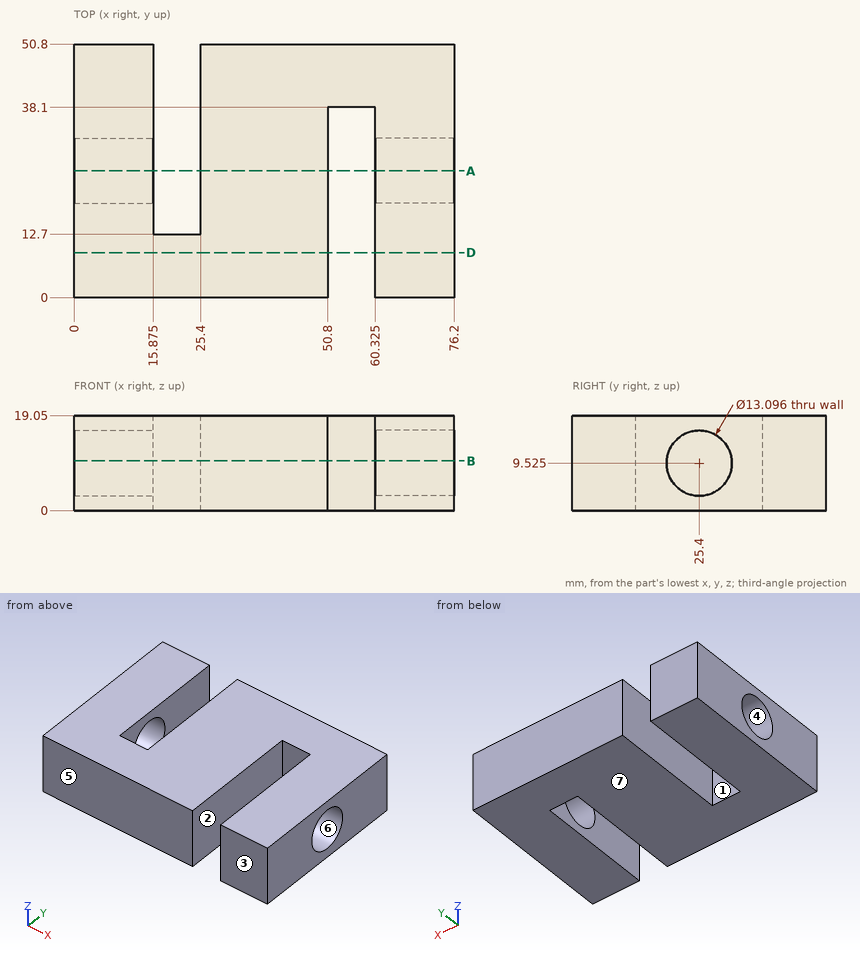
Verification items for this drawing (mm, ordinates from the low corner). A direction names the side the tool comes from. Give positions to 0.01 mm unless a question says otherwise; leave off trailing zeros. Write each loop counter-clockwise with the first axis right and the second up, starting at its lowest first coordinate (ties: lowest second). Pieces come first, ordered by that corner, then holes. Notation, with made-up numbers: M -26,-0.75 L 33,-0.75 A5 cw 33,8.25 Z; hole C 40.5,3.5 d3. An arc over 180 degrees is marked long. Use one line per item in the form item = value.
(1) Tool access check on the marked faces 1, 2 and 3. Record the directions out of +Z, -Z, +X, -X, +Y, -Y that give a thin tool (end or side, any length) a straight path to the whole face; none if there is none.
Answer block:
face_1 = +Z, -Z, +Y
face_2 = +Z, -Z, -Y
face_3 = +Z, -Z, +X, -X, -Y
(2) Section check D-D on y = 9. Record the boundary of the cut face in (x, z) (3 decimals).
Answer block:
outline = M 0,0 L 50.8,0 L 50.8,19.05 L 0,19.05 Z; M 60.325,0 L 76.2,0 L 76.2,19.05 L 60.325,19.05 Z
(3) Section check B-B on z = 10. Record the boundary of the cut face in (x, y) (1 decimal).
Answer block:
outline = M 0,0 L 50.8,0 L 50.8,38.1 L 60.3,38.1 L 60.3,31.9 L 76.2,31.9 L 76.2,50.8 L 25.4,50.8 L 25.4,12.7 L 15.9,12.7 L 15.9,18.9 L 0,18.9 Z; M 0,31.9 L 15.9,31.9 L 15.9,50.8 L 0,50.8 Z; M 60.3,0 L 76.2,0 L 76.2,18.9 L 60.3,18.9 Z
(4) Section check A-A on y = 25.4. State how many separate pieces and enclosed holes the cut face has, plus the area to 3 significant figures.
Answer block:
separate_pieces = 5
enclosed_holes = 0
area = 673 mm2
(5) Material ranges on line 1 along X through (y, z) = (15, 3.25) (3 decimals); line 2 along X through (y, z) = (8, 4) (3 decimals); line 3 along X through (y, z) = (43, 4.5) (3 decimals), recorded low to high.
Answer block:
line_1 = 0 to 15.875, 25.4 to 50.8, 60.325 to 76.2
line_2 = 0 to 50.8, 60.325 to 76.2
line_3 = 0 to 15.875, 25.4 to 76.2
(6) Draft check along Y on the marked faces 4, 5, 6 and 7. Enter one of: pulls with the +Y half, pulls with the -Y half, needs draft (parallel to the pull), parting line crosses it, or undercut.
Answer block:
face_4 = undercut
face_5 = pulls with the -Y half
face_6 = undercut
face_7 = needs draft
(7) Depth check by flat-ended pin: P1, Ø8, axis at y = 25.4, z = 9.525, coming from the -X side; P2, Ø4, axis at x = 58, z = 2.5, coming from the -Y side. Enter the tip coordinate at first touch or a pass-through.
Answer block:
P1 = 25.4
P2 = 38.1
